Design review of the part built by this model. Coordinates are the model's own, in mm. Face numbers are marked on the shaded views. A direction names the side the tool comes from. Coordinates: 2 decimals unless noted, no trailing zeros. Order: outer loops, then holes, each group sorted by start corner. A loop starts at its lowest first (then second) coordinate and runs counter-clockwise, first axis right, second up. Notation, with made-up numbers: M 18,11 L 54,11 A6 ccw 54,16 Z; hole C 80.25,75 d8. An arc over 180 degrees is marked long. Use CSV: the item, a comma, the result in double quotes.
```python
from build123d import *

# Parameters (mm, degrees)
F1_DEPTH      = 5
F2_DEPTH      = 19.05
F3_DEPTH      = 5
F4_W          = 12.7
F4_H          = 1.5
F5_DEPTH      = 37.23736246
F5_DEPTH_BACK = 7.25
F6_START      = 18.6339281499
F6_DEPTH      = 1.5
F7_START      = 18.6339281499
F7_DEPTH      = 6.3660718501


with BuildPart() as f1:
    # F0 (on Top) → F1 (new body)
    with BuildSketch(Plane.XY):
        Polygon((-34.23736246, 9.9433793599), (-34.23736246, 6.9433793599), (-16.73736246, 6.9433793599), (-16.73736246, -20.0566206401), (-34.23736246, -20.0566206401), (-34.23736246, -23.0566206401), (-13.73736246, -23.0566206401), (-13.73736246, 9.9433793599), align=None)
    extrude(amount=F1_DEPTH)

    # F0 (on Top) → F2 (join)
    with BuildSketch(Plane.XY):
        Polygon((-34.23736246, -20.0566206401), (-34.23736246, -9.6503041635), (-37.23736246, -9.6503041635), (-37.23736246, -23.0566206401), (-34.23736246, -23.0566206401), align=None)
    extrude(amount=F2_DEPTH)

    # F0 (on Top) → F3 (join)
    with BuildSketch(Plane.XY):
        Polygon((-34.23736246, -9.6503041635), (-34.23736246, 6.9433793599), (-34.23736246, 9.9433793599), (-37.23736246, 9.9433793599), (-37.23736246, -9.6503041635), align=None)
    extrude(amount=F3_DEPTH)

    # F4 (on Right) → F5 (join, two sides)
    with BuildSketch(Plane.YZ) as f5_sk:
        with Locations((-16.7916113675, 19.3839281499)):
            Rectangle(F4_W, F4_H)
    extrude(amount=-F5_DEPTH)
    extrude(f5_sk.sketch, amount=F5_DEPTH_BACK)

    # F0 (on Top) → F6 (join)
    with BuildSketch(Plane.XY.offset(F6_START)):
        with BuildLine():
            Line((2.0767554697, -8.3933884358), (2.0767554697, -1.3145332665))
            ThreePointArc((2.0767554697, -1.3145332665), (0.5588870059, -2.6728853277), (-0.9137062697, -1.2655779555))
            Line((-0.9137062697, -1.2655779555), (-0.9137062697, -8.3933884358))
            Line((-0.9137062697, -8.3933884358), (-0.9137062697, -23.0566206401))
            Line((-0.9137062697, -23.0566206401), (2.0767554697, -23.0566206401))
            Line((2.0767554697, -23.0566206401), (2.0767554697, -8.3933884358))
        make_face()
    extrude(amount=F6_DEPTH)

    # F0 (on Top) → F7 (join)
    with BuildSketch(Plane.XY.offset(F7_START)):
        with BuildLine():
            Line((2.0767554697, -1.3145332665), (2.0767554697, -1.0316392973))
            ThreePointArc((2.0767554697, -1.0316392973), (0.5588870059, 0.3267127639), (-0.9137062697, -1.0805946084))
            Line((-0.9137062697, -1.0805946084), (-0.9137062697, -1.2655779555))
            ThreePointArc((-0.9137062697, -1.2655779555), (0.5588870059, -2.6728853277), (2.0767554697, -1.3145332665))
        make_face()
    extrude(amount=F7_DEPTH)


solid = f1.part
```
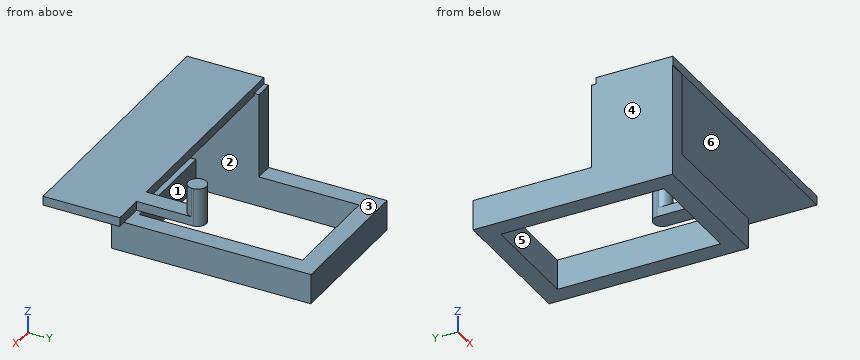
(1) Add section A-A on y = -12.5. State the section outline as (x, z) points, and give its area (3 significant figures).
The answers:
outline,"M -37.24,0 L -34.24,0 L -34.24,18.63 L 7.25,18.63 L 7.25,20.13 L -37.24,20.13 Z; M -16.74,0 L -13.74,0 L -13.74,5 L -16.74,5 Z"
area,"138 mm2"
(2) For the marked faces 1, 2 and 3, list the 3-axis set-ups (+Z, -Z, +X, -X, +Y, -Y) from which the entire face can be reached by the end or side of a thin tool; tool diameter is ignored.
The answers:
face 1,"-Z"
face 2,"none"
face 3,"+X, +Y"
(3) Clearance check with flat-ended pins moving along their axes: P1, Ø12, axis at x = -18, y = -3.5, coming from the +Z side; P2, Ø7, axis at y = -6, z = 21.5, coming from the +X side; P3, Ø4, axis at y = -10, z = 2, coming from the +X side; P4, Ø10, axis at x = -31, y = -5.5, coming from the -Z side. State where each tip first meets the part, or that it passes through.
The answers:
P1,"stops at z = 5"
P2,"stops at x = 2.08"
P3,"stops at x = -13.74"
P4,"stops at z = 0"
(4) Add section B-B on x = -30.5. State the section outline as (y, z) points, and give its area (4 significant figures).
The answers:
outline,"M -23.14,18.63 L -10.44,18.63 L -10.44,20.13 L -23.14,20.13 Z; M -23.06,0 L -20.06,0 L -20.06,5 L -23.06,5 Z; M 6.94,0 L 9.94,0 L 9.94,5 L 6.94,5 Z"
area,"49.05 mm2"
(5) The part is to be moulded in two halves that separate along X. For the marked faces 4, 5 and 6, say which applies: pulls with the +X half, pulls with the -X half, needs draft (parallel to the pull), parting line crosses it, or undercut.
The answers:
face 4,"pulls with the -X half"
face 5,"undercut"
face 6,"needs draft"
(6) Add section C-C on y = -7. State the section outline as (x, z) points, and give its area (3 significant figures).
The answers:
outline,"M -37.24,0 L -34.24,0 L -34.24,5 L -37.24,5 Z; M -16.74,0 L -13.74,0 L -13.74,5 L -16.74,5 Z; M -0.91,18.63 L 2.08,18.63 L 2.08,20.13 L -0.91,20.13 Z"
area,"34.5 mm2"
(7) Add section D-D on y = 2. State the section outline as (x, z) points, and give its area (3 significant figures).
The answers:
outline,"M -37.24,0 L -34.24,0 L -34.24,5 L -37.24,5 Z; M -16.74,0 L -13.74,0 L -13.74,5 L -16.74,5 Z"
area,"30.0 mm2"
(8) Wall thickness on probe 1 along X at (y, z) = (-19, 3); probe 2 along X at (y, z) = (-13, 7.5); probe 3 along Z at (x, y) = (1.5, -2): over which ranges is each line inside the solid? List them lowest first.
The answers:
probe 1,"x = -37.24 to -34.24, -16.74 to -13.74"
probe 2,"x = -37.24 to -34.24"
probe 3,"z = 18.63 to 25"
